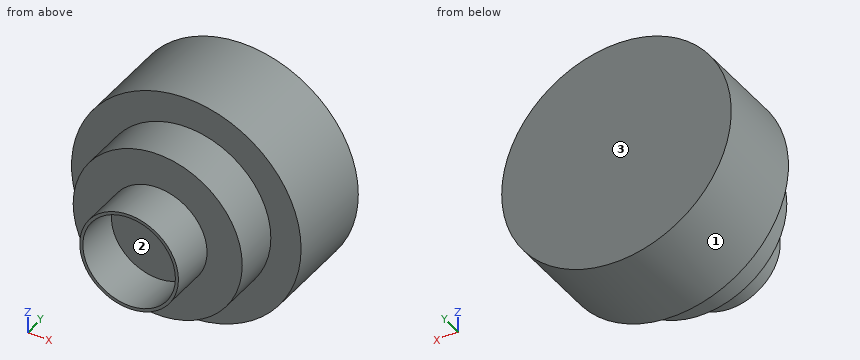
```python
from build123d import *

# Parameters (mm, degrees)
F0_R     = 31
F1_DEPTH = 12.5
F2_R     = 22.832123
F3_DEPTH = 25
F4_R     = 13.330594
F4_R_2   = 12.5
F5_DEPTH = 12.5


with BuildPart() as f1:
    # F0 (on Front) → F1 (new body, symmetric)
    with BuildSketch(Plane.XZ):
        Circle(F0_R)
    extrude(amount=F1_DEPTH, both=True)

    # F2 (on Front) → F3 (join)
    with BuildSketch(Plane.XZ):
        Circle(F2_R)
    extrude(amount=F3_DEPTH)

    # F4 (on face) → F5 (join, symmetric)
    with BuildSketch(Plane.XZ.offset(25)):
        Circle(F4_R)
        Circle(F4_R_2, mode=Mode.SUBTRACT)
    extrude(amount=F5_DEPTH, both=True)


solid = f1.part
```
Input: part model. Units: mm. Frame: model coordinates. Face numbers are marked on the shaded views. Round coordinates to 2 decimals unless told otherwise and drop trailing zeros. Loops run counter-clockwise (first coordinate to the right, second up) from the corner with the lowest first, then second, coordinate; pieces in that order, holes last. Notation, with made-up numbers: (-11, 67) -> (34, 67) arc R8 ccw to (34, 71) -> close; hole circle Ø8 at (-1, 19). An arc over 180 degrees is marked (long way). One line per item, written item: value.
(1) Material intervals for line 1 (Z direction, x = 0, y = -30.75); line 2 (Y direction, x = 28, z = -3); line 3 (Y direction, x = -2.5, z = 14), sorted ascending. Write a range as [from, to].
Geometry check:
line 1: [-13.33, -12.5], [12.5, 13.33]
line 2: [-12.5, 12.5]
line 3: [-25, 12.5]
(2) Pin query (flat end, axial travel): pin 1 (6 mm diameter, centred on x = -20, y = 2, fed in from +Z); pin 2 (6 mm diameter, centred on x = 8.5, y = -0.5, fed in from +Z); pin 3 (5 mm diameter, centred on x = 0, y = -5, fed in from -Z); pin 4 (20 mm diameter, centred on x = 4, z = 3.5, fed in from -Y). Return the tip coordinate at first contact, or that it passes through.
Geometry check:
pin 1: z = 25.92
pin 2: z = 30.51
pin 3: z = -31
pin 4: y = -37.5
(3) Section B-B (x = 0). Return the cut outline in (y, z).
Geometry check:
outline: (-37.5, -13.33) -> (-25, -13.33) -> (-25, -22.83) -> (-12.5, -22.83) -> (-12.5, -31) -> (12.5, -31) -> (12.5, 31) -> (-12.5, 31) -> (-12.5, 22.83) -> (-25, 22.83) -> (-25, 13.33) -> (-37.5, 13.33) -> (-37.5, 12.5) -> (-25, 12.5) -> (-25, -12.5) -> (-37.5, -12.5) -> close
(4) Section A-A (z = 0). Return the cut outline in (x, y), plus the area to 3 significant figures.
Geometry check:
outline: (-31, -12.5) -> (-22.83, -12.5) -> (-22.83, -25) -> (-13.33, -25) -> (-13.33, -37.5) -> (-12.5, -37.5) -> (-12.5, -25) -> (12.5, -25) -> (12.5, -37.5) -> (13.33, -37.5) -> (13.33, -25) -> (22.83, -25) -> (22.83, -12.5) -> (31, -12.5) -> (31, 12.5) -> (-31, 12.5) -> close
area: 2,140 mm2
(5) Mould query, pull axis X, two halves, no side actions, for the marked faces 1, 2 and 3. Classes: pulls with the +X half, pulls with the -X half, needs draft (parallel to the pull), parting line crosses it, or undercut.
Geometry check:
face 1: parting line crosses it
face 2: undercut
face 3: needs draft
(6) Section D-D (y = -7). Return the cut outline in (x, z).
Geometry check:
outline: circle Ø62 at (0, 0)
(7) Section C-C (y = -27). Return the cut outline in (x, z), plus the area to 3 significant figures.
Geometry check:
outline: circle Ø26.66 at (0, 0); hole circle Ø25 at (0, 0)
area: 67.4 mm2
